```python
from build123d import *

# Parameters (mm, degrees)
SKETCH1_W           = 40
SKETCH1_H           = 16
BOSS_EXTRUDE1_DEPTH = 1.6
SKETCH2_R           = 1.75
CUT_EXTRUDE1_DEPTH  = 1.6
BOSS_EXTRUDE2_DEPTH = 5.7
SKETCH4_W           = 7
SKETCH4_H           = 12.6
BOSS_EXTRUDE3_DEPTH = 5.7


with BuildPart() as part:
    # Sketch1 → Boss-Extrude1 (new body)
    with BuildSketch(Plane(origin=(0, 0, 0), x_dir=(1, 0, 0), z_dir=(0, 1, 0))):
        Rectangle(SKETCH1_W, SKETCH1_H)
    extrude(amount=BOSS_EXTRUDE1_DEPTH)

    # Sketch2 → Cut-Extrude1 (cut)
    with BuildSketch(Plane(origin=(0, 0, 0), x_dir=(1, 0, 0), z_dir=(0, 1, 0))):
        with Locations(Location((-17, 5, 0), (0, 0, 270))):
            Circle(SKETCH2_R)
        with Locations(Location((-17, -5, 0), (0, 0, 270))):
            Circle(SKETCH2_R)
        with Locations(Location((-2.5, 5, 0), (0, 0, 270))):
            Circle(SKETCH2_R)
        with Locations(Location((17, 5, 0), (0, 0, 270))):
            Circle(SKETCH2_R)
    extrude(amount=CUT_EXTRUDE1_DEPTH, mode=Mode.SUBTRACT)

    # Sketch3 → Boss-Extrude2 (add)
    with BuildSketch(Plane(origin=(0, 1.6, 0), x_dir=(1, 0, 0), z_dir=(0, 1, 0))):
        Polygon((0.9, 7.5), (16.2, 12.5), (17.2, 12.5), (1.9, 7.5), (13.7, 7.5), (13.7, -0.5), (0.9, -0.5), align=None)
    extrude(amount=BOSS_EXTRUDE2_DEPTH)

    # Sketch4 → Boss-Extrude3 (add)
    with BuildSketch(Plane(origin=(0, 1.6, 0), x_dir=(1, 0, 0), z_dir=(0, 1, 0))):
        with Locations((-12.9, 0)):
            Rectangle(SKETCH4_W, SKETCH4_H)
    extrude(amount=BOSS_EXTRUDE3_DEPTH)


solid = part.part
```
Input: part model. Units: mm. Frame: model coordinates. A direction names the side the tool comes from. Coordinates: 2 decimals unless noted, no trailing zeros. Loops run counter-clockwise (first coordinate to the right, second up) from the corner with the lowest first, then second, coordinate; pieces in that order, holes last. Notation, with made-up numbers: M 45,42 L 80,42 A28 cw 80,78 Z; hole C 84,-37.5 d7. An arc over 180 degrees is marked long. One line per item, written item: value.
(1) Pin query (flat end, axial travel): pin 1 (1.5 mm diameter, centred on y = 3.5, z = 4.5, fed in from +X); pin 2 (0.8 mm diameter, centred on x = -6.5, y = 1, fed in from -Z); pin 3 (0.6 mm diameter, centred on x = -16, z = -5, fed in from -Y). Return the tip coordinate at first contact, or that it passes through.
Filled in:
pin 1: x = -9.4
pin 2: z = -8
pin 3: y = 1.6
(2) Pull-direction query (Z, two-part tool) for faces 1 (the cylindrical face through (18.735, 0.789, -5.228)), 2 (the flat face through (13.7, 4, -4)), 3 (the flat face through (-13, 4, 6.3)); classes: +Z half, -Z half, draft (parallel to the pull), parting line (faces both ways), or undercut.
Filled in:
face 1: undercut
face 2: draft
face 3: +Z half
(3) Line query: line 1 along Z through (x, y) = (-17, 1); line 2 along X through (y, z) = (1.3, -5); line 3 along X through (y, z) = (1.75, -5.75). Output: solid intervals per line, ascending. Write a range as from..to.
Filled in:
line 1: -8..-6.75, -3.25..3.25, 6.75..8
line 2: -20..-18.75, -15.25..-4.25, -0.75..15.25, 18.75..20
line 3: -16.4..-9.4, 0.9..13.7
(4) Section C-C (z = 5). Output: boundary loops of the cut face in (x, y).
Filled in:
outline: M -20,0 L -18.75,0 L -18.75,1.6 L -20,1.6 Z; M -16.4,1.6 L -15.25,1.6 L -15.25,0 L 20,0 L 20,1.6 L -9.4,1.6 L -9.4,7.3 L -16.4,7.3 Z
(5) Reachability of faces 4 (the flat face through (9.85, 1.6, -10.26)), 5 (the flat face through (-16.4, 4, 0)), 6 (the flat face through (0.9, 4, -3)), 7 (the cylindrical face through (-15.265, 0.789, -5.228)), 8 (the flat face through (8, 4, -7.5)) from +Z, -Z, +X, -X, +Y, -Y: full face, straight path, thin tool, end or side. Return the list, or none.
Filled in:
face 4: -Z, +X, -X, -Y
face 5: +Z, -Z, -X, +Y
face 6: +Z, -Z, +Y
face 7: -Y
face 8: +X, +Y
(6) Section A-A (y = 2). Output: boundary loops of the cut face in (x, z).
Filled in:
outline: M -16.4,-6.3 L -9.4,-6.3 L -9.4,6.3 L -16.4,6.3 Z; M 0.9,-7.5 L 16.2,-12.5 L 17.2,-12.5 L 1.9,-7.5 L 13.7,-7.5 L 13.7,0.5 L 0.9,0.5 Z
(7) Section B-B (x = -2.5). Output: boundary loops of the cut face in (y, z), and give its area (3 significant figures).
Filled in:
outline: M 0,-8 L 1.6,-8 L 1.6,-6.75 L 0,-6.75 Z; M 0,-3.25 L 1.6,-3.25 L 1.6,8 L 0,8 Z
area: 20.0 mm^2
(8) Section D-D (x = -17). Output: boundary loops of the cut face in (y, z).
Filled in:
outline: M 0,-8 L 1.6,-8 L 1.6,-6.75 L 0,-6.75 Z; M 0,-3.25 L 1.6,-3.25 L 1.6,3.25 L 0,3.25 Z; M 0,6.75 L 1.6,6.75 L 1.6,8 L 0,8 Z
